```python
from build123d import *

# Parameters (mm, degrees)
SKETCH1_W           = 26.035
SKETCH1_H           = 42.7228
BOSS_EXTRUDE1_DEPTH = 25.4
SKETCH19_R          = 6.35
CUT_EXTRUDE1_DEPTH  = 31.75


with BuildPart() as part:
    # Sketch1 → Boss-Extrude1 (new body)
    with BuildSketch(Plane.XY):
        Rectangle(SKETCH1_W, SKETCH1_H)
    extrude(amount=BOSS_EXTRUDE1_DEPTH)

    # Sketch19 → Cut-Extrude1 (cut)
    with BuildSketch(Plane(origin=(5.123678059, 23.111418192, 0), x_dir=(-0.976296007, 0.216439614, 0), z_dir=(-0.216439614, -0.976296007, 0))):
        with Locations((1.439519896, -12.397187114)):
            Circle(SKETCH19_R)
    extrude(amount=CUT_EXTRUDE1_DEPTH, mode=Mode.SUBTRACT)


solid = part.part
```
Build history of the part. All positions in model axes, mm. A direction names the side the tool comes from. Round coordinates to 2 decimals unless told otherwise and drop trailing zeros. Write each loop counter-clockwise with the first axis right and the second up, starting at its lowest first coordinate (ties: lowest second). Pieces come first, ordered by that corner, then holes.
1) 3-axis set-ups, long thin cutter, end or side, ignore diameter. For faces 1 (the flat face through (0, -21.361, 13)), 2 (the flat face through (-3.067, -7.594, 12.308)): which of +Z, -Z, +X, -X, +Y, -Y reach the whole face in a straight line?
2) Band-saw the part on B-B, the plane z = 15. List the corners of the cut face in (x, y).
3) Drill centre lines: probe 1 along Z at (x, y) = (0.25, 7); probe 2 along X at (y, z) = (-3.5, 18); probe 3 along Z at (x, y) = (-0.5, -4). Where is each one in solid material? Low to high.
4) Band-saw the part on A-A, the plane z = 8. List the corners of the cut face in (x, y).
5) Mould opens along Y. For faces 3 (the flat face through (-3, 21.361, 15)), 4 (the cylindrical face through (6.461, 6.485, 12.118)), 5 (the flat face through (-13.018, 0, 13)) say: +Y half, -Y half, draft (parallel to the pull), parting line (faces both ways), or undercut.
6) Pin check, flat tip, straight feed: pin 1 (10 mm diameter, centred on x = 3, z = 14.5, fed in from +Y). Stop position of the tip, or through.
Ans:
1. face 1: +Z, -Z, +X, -X, -Y
1. face 2: none
2. outline: (-13.02, -21.36) - (13.02, -21.36) - (13.02, 21.36) - (9.19, 21.36) - (2.5, -8.83) - (-8.81, -6.32) - (-2.67, 21.36) - (-13.02, 21.36) - close
3. probe 1: z = 0 to 6.05, 18.74 to 25.4
3. probe 2: x = -13.02 to -5.31, 0.81 to 13.02
3. probe 3: z = 0 to 6.31, 18.48 to 25.4
4. outline: (-13.02, -21.36) - (13.02, -21.36) - (13.02, 21.36) - (7.95, 21.36) - (1.32, -8.57) - (-7.63, -6.58) - (-1.43, 21.36) - (-13.02, 21.36) - close
5. face 3: +Y half
5. face 4: undercut
5. face 5: draft
6. pin 1: stops at y = 21.36
